Autodesk Inventor part; units mm, degrees
ref_plane "YZ Plane" through (0, 0, 0) normal (1, 0, 0) x (0, 1, 0)
ref_plane "XZ Plane" through (0, 0, 0) normal (0, 1, 0) x (-1, 0, 0)
ref_plane "XY Plane" through (0, 0, 0) normal (0, 0, 1) x (1, 0, 0)
sketch "Sketch1" plane through (0, 0, 0) normal (0, 0, 1) x (1, 0, 0)
  circle A0 centre (0, 0) radius 10
  circle A1 centre (0, 0) radius 11.2
  circle A2 centre (0, 0) radius 15.75
  dimension "d0" = 20
  dimension "d1" = 1.2
  dimension "d12" = 31.5
  dimension "d16" = 22.4
extrude "Extrusion1" add sketch "Sketch1" against normal blind 31.2 contours A0 | A1 | A2
extrude "Extrusion2" add sketch "Sketch1" along normal blind 80 contours A1
sketch "Sketch2" plane through (0, 0, 0) normal (0, 1, 0) x (-1, 0, 0)
  line L0 (-15.75, -31.2) -> (15.75, -31.2)
  line L1 (15.75, 0) -> (-15.75, 0) construction
  line L2 (-15.75, -31.2) -> (15.75, -31.2)
  line L3 (15.75, 0) -> (-15.75, 0)
  line L4 (15.75, -31.2) -> (15.75, 0) construction
  line L5 (-15.75, -31.2) -> (-15.75, 0) construction
  line L6 (-15.75, 0) -> (-15.75, -31.2) construction
  line L7 (15.75, -1.2) -> (-15.75, -1.2)
  line L8 (15.75, -1.2) -> (15.75, -31.2)
  line L9 (-15.75, -1.2) -> (-15.75, -31.2)
  line L10 (15.75, 0) -> (15.75, -31.2)
  arc A0 (15.75, -1.2) -> (12.9532, -3.1146) centre (15.75, -4.2) ccw
  arc A1 (-12.9532, -3.1146) -> (-15.75, -1.2) centre (-15.75, -4.2) ccw
  arc A2 (-2.7968, -29.2854) -> (2.7968, -29.2854) centre (0, -28.2) ccw
  line L11 (2.7968, -29.2854) -> (12.9532, -3.1146)
  line L12 (-12.9532, -3.1146) -> (-2.7968, -29.2854)
  line L13 (0, -31.2) -> (0, -1.2)
  line L14 (-11.2, 0) -> (-11.2, 80) construction
  line L15 (-15.75, 0) -> (-11.2, 4.55)
  line L16 (-11.2, 0) -> (-11.2, 80)
  line L17 (-11.2, 4.55) -> (-11.2, 0)
  line L18 (-11.2, 0) -> (-15.75, 0)
  point P0 (0, 0)
  dimension "d7" = 1.2
  dimension "d10" = 3
  dimension "d14" = 45
revolve "Revolution1" cut sketch "Sketch2" angle 360 about axis through (0, 0, -31.2) along (0, 0, 1) contours L9 A1 L12 A2 L0
revolve "Revolution2" add sketch "Sketch2" angle 360 about axis through (0, 0, -31.2) along (0, 0, 1) contours L3 L15 L16 | A2 L12 A1 L7 L13
properties part number "Marker Barrel" material "ABS Plastic"
Part model, mm, in its own coordinate system. A direction names the side the tool comes from. Round coordinates to 2 decimals unless told otherwise and drop trailing zeros. Order: outer loops, then holes, each group sorted by start corner. A loop starts at its lowest first (then second) coordinate and runs counter-clockwise, first axis right, second up. Notation, with made-up numbers: M 10.25,82.25 L 57.25,82.25 A19 cw 57.25,106.25 Z; hole C 27,80.5 d10. An arc over 180 degrees is marked long. Put each result on its own line as item: value. Start each with the question number.
1. Tool access for faces 4 (the face through (-2.05, 15.616, -0.592)), 5 (the face through (-2.17, 9.76, 39.44)): list every direction of +Z, -Z, +X, -X, +Y, -Y with a clear straight run to the whole face (end or side of a thin tool).
2. Drop flat-ended pins along their axis: pin 1 (12 mm diameter, centred on y = 12, z = 29, fed in from +X); pin 2 (2 mm diameter, centred on x = -4, z = 10, fed in from +Y); pin 3 (2 mm diameter, centred on x = -7, z = 64.5, fed in from -Y). Give the stop position or say it passes through.
3. Slice it at D-D on z = -8. List the corners of the cut face in (x, y), then the cut area to 3 significant figures.
4. Drill centre lines: probe 1 along Y at (x, z) = (0, 31); probe 2 along X at (y, z) = (-0.5, 37); probe 3 along X at (y, z) = (5.5, 53.5). Where is each one in solid material? Low to high. Write a range as [from, to].
5. Slice it at C-C on z = 47. List the corners of the cut face in (x, y).
6. Two-plate mould, pull along X, no slides. Class faces 1 (the face through (-8, 7, 80)), 2 (the face through (-11.19, -0.49, 41.75)), 3 (the face through (0, 0, 0)): +X half, -X half, draft (parallel to the pull), parting line (faces both ways), or undercut.
7. Slice it at A-A on x = 0. List the corners of the cut face in (y, z).
Findings:
1. face 4: +Z, -Z
1. face 5: +Z
2. pin 1: x = 9.46
2. pin 2: y = 10.79
2. pin 3: y = -9.46
3. outline: C 0,0 d22.11
3. area: 384 mm2
4. probe 1: [-11.2, -10], [10, 11.2]
4. probe 2: [-11.19, -9.99], [9.99, 11.19]
4. probe 3: [-9.76, -8.35], [8.35, 9.76]
5. outline: C 0,0 d22.4; hole C 0,0 d20
6. face 1: draft
6. face 2: parting line
6. face 3: undercut
7. outline: M -15.75,-1.2 A3 cw -12.95,-3.11 L -2.8,-29.29 A3 ccw 2.8,-29.29 L 12.95,-3.11 A3 cw 15.75,-1.2 L 15.75,0 L 11.2,4.55 L 11.2,80 L 10,80 L 10,0 L -10,0 L -10,80 L -11.2,80 L -11.2,4.55 L -15.75,0 Z
